Verification items for the finished model (mm, model axes). Face numbers are marked on the shaded views. A direction names the side the tool comes from. Coordinates: 2 decimals unless noted, no trailing zeros. Loops run counter-clockwise (first coordinate to the right, second up) from the corner with the lowest first, then second, coordinate; pieces in that order, holes last. Notation, with made-up numbers: (7, 43) - (28, 43) arc R20 cw to (28, 55) - close; hole circle Ø11 at (62.25, -39.75). An arc over 180 degrees is marked (long way). Answer as CSV lines item,"result". Start each with the question number.
1. Cross-section at C-C (z = -48). Enter the section's corners in (x, y) (3 decimals).
2. Set-up check for the marked faces 1 and 2: record each of +Z, -Z, +X, -X, +Y, -Y from which the full face is reachable in a straight line by a thin tool's end or side.
3. Gauge pin test, flat ends, axial feed: P1, Ø4, axis at y = 9, z = -36.5, coming from the -X side; P2, Ø3, axis at y = 14, z = -23.5, coming from the +X side; P3, Ø7.5, axis at y = 31, z = -40, coming from the +X side. Record the tip position at first contact, or that the pin passes through.
4. Cross-section at B-B (x = 13). Enter the section's corners in (y, z) (3 decimals).
5. Release check for a two-part mould opening along Y. For the marked faces 3, 4, 5 and 6 record: pulls with the +Y half, pulls with the -Y half, needs draft (parallel to the pull), parting line crosses it, or undercut.
6. Cross-section at D-D (x = 60). Enter the section's corners in (y, z) (3 decimals), plus the area to 3 significant figures.
7. Material ranges on line 1 (X direction, y = 3.5, z = -13.5) (3 decimals); line 2 (X direction, y = 24.5, z = -34) (3 decimals); line 3 (Y direction, x = 59.5, z = -27.5) (3 decimals), recorded low to high. Write a range as [from, to].
8. Cross-section at A-A (z = -28). Enter the section's corners in (x, y) (3 decimals).
```python
from build123d import *

# Parameters (mm, degrees)
SKETCH1_W           = 79.375
SKETCH1_H           = 57.14999999999999
BASE_EXTRUDE_DEPTH  = 9.525
SKETCH2_R           = 5.1562
CUT_EXTRUDE1_DEPTH  = 99.27125088244273
BOSS_EXTRUDE1_DEPTH = 11.112499999999999
FILLET1_R           = 4.7625
FILLET3_R           = 3.175
FILLET5_R           = 6.35
FILLET6_R           = 3.175


with BuildPart() as part:
    # Sketch1 → Base-Extrude (new body)
    with BuildSketch(Plane(origin=(0, 0, 0), x_dir=(1, 0, 0), z_dir=(0, 1, 0))):
        with Locations((39.6875, 28.574999999999996)):
            Rectangle(SKETCH1_W, SKETCH1_H)
    extrude(amount=BASE_EXTRUDE_DEPTH)

    # Sketch2 → Cut-Extrude1 (cut, through all)
    with BuildSketch(Plane(origin=(0, 9.525, 0), x_dir=(-1, 0, 0), z_dir=(0, 1, 0))):
        with Locations(Location((-11.112499999999999, -46.037499999999994, 0), (0, 0, 90))):
            Circle(SKETCH2_R)
        with Locations(Location((-11.112499999999999, -11.112499999999997, 0), (0, 0, 90))):
            Circle(SKETCH2_R)
        with Locations(Location((-68.2625, -11.112499999999997, 0), (0, 0, 90))):
            Circle(SKETCH2_R)
        with Locations(Location((-68.2625, -46.037499999999994, 0), (0, 0, 90))):
            Circle(SKETCH2_R)
    extrude(amount=-CUT_EXTRUDE1_DEPTH, mode=Mode.SUBTRACT)

    # Sketch3 → Boss-Extrude1 (add, symmetric)
    with BuildSketch(Plane(origin=(39.6875, 0, 0), x_dir=(0, 0, -1), z_dir=(1, 0, 0))):
        with BuildLine():
            Line((15.081249999999999, 9.525), (57.15, 9.525))
            Line((57.15, 9.525), (45.642080901347875, 34.2124833053063))
            ThreePointArc((45.642080901347875, 34.2124833053063), (40.65983135726152, 39.74024710013013), (33.435990911126424, 41.52773480629668))
            Line((33.435990911126424, 41.52773480629668), (24.475888920836205, 41.03647902618064))
            ThreePointArc((24.475888920836205, 41.03647902618064), (22.228971581677126, 38.79627321294108), (24.202681662531663, 36.31199703436931))
            Line((24.202681662531663, 36.31199703436931), (28.991955012405008, 35.48840889689211))
            ThreePointArc((28.991955012405008, 35.48840889689211), (34.924994788062534, 28.439370658797703), (28.97494247235726, 21.40468669276046))
            Line((28.97494247235726, 21.40468669276046), (17.72572001228568, 19.498181673786302))
            ThreePointArc((17.72572001228568, 19.498181673786302), (15.830857484241669, 18.416745811263993), (15.081249999999997, 16.367820203902035))
            Line((15.081249999999997, 16.367820203902035), (15.081249999999999, 9.525))
        make_face()
    extrude(amount=BOSS_EXTRUDE1_DEPTH, both=True)

    # Fillet1
    fillet1_edges = [part.edges().sort_by_distance(p)[0] for p in [
        (0, 4.7625, -57.15),
        (79.375, 4.7625, -57.15),
        (79.375, 4.7625, 0),
        (0, 4.7625, 0),
    ]]
    fillet(fillet1_edges, radius=FILLET1_R)

    # Fillet3
    fillet3_edges = [part.edges().sort_by_distance(p)[0] for p in [
        (16.668750000000003, 9.525, -57.15),
        (39.6875, 9.525, 0),
        (0, 9.525, -28.575),
        (79.375, 9.525, -28.575),
        (62.70625, 9.525, -57.15),
        (77.98009604540093, 9.525, -55.75509604540093),
        (1.3949039545990662, 9.525, -55.75509604540093),
        (77.98009604540093, 9.525, -1.3949039545990662),
        (1.3949039545990667, 9.525, -1.3949039545990662),
    ]]
    fillet(fillet3_edges, radius=FILLET3_R)

    # Fillet5
    # the kernel refuses this fillet: 6.35 mm, written as the material it adds along each edge
    with BuildSketch(Plane(origin=(28.575000000000003, 9.525, -15.081249999999997), x_dir=(-1, 0, 0), z_dir=(0, 0, -1))) as fillet5_piece_1:
        with BuildLine():
            CenterArc((FILLET5_R, FILLET5_R), FILLET5_R, 180, 90)
            Line((0, FILLET5_R), (0, 0))
            Line((0, 0), (FILLET5_R, 0))
        make_face()
    extrude(amount=38.893750000000004)
    with BuildSketch(Plane(origin=(50.8, 9.525, -15.081249999999999), x_dir=(0, 0, 1), z_dir=(-1, 0, 0))) as fillet5_piece_2:
        with BuildLine():
            CenterArc((FILLET5_R, FILLET5_R), FILLET5_R, 180, 90)
            Line((3.55e-15, FILLET5_R), (0, 0))
            Line((0, 0), (FILLET5_R, 0))
        make_face()
    extrude(amount=22.224999999999994)
    with BuildSketch(Plane(origin=(50.8, 9.525, -15.081249999999997), x_dir=(1, 0, 0), z_dir=(0, 0, -1))) as fillet5_piece_3:
        with BuildLine():
            CenterArc((FILLET5_R, -FILLET5_R), FILLET5_R, 90, 90)
            Line((0, -FILLET5_R), (0, 0))
            Line((0, 0), (FILLET5_R, 0))
        make_face()
    extrude(amount=38.893750000000004)
    with BuildSketch(Plane(origin=(28.575000000000003, 6.350000000000001, -53.975), x_dir=(0, 1, 0), z_dir=(0, 0, 1))) as fillet5_piece_4_section:
        with BuildLine():
            CenterArc((3.174999999999999 + FILLET5_R, FILLET5_R), FILLET5_R, 180.00000000000003, 90)
            Line((3.174999999999999, FILLET5_R), (3.174999999999999, 0))
            Line((3.174999999999999, 0), (3.174999999999999 + FILLET5_R, 0))
        make_face()
    fillet5_piece_4 = revolve(axis=Axis((28.575000000000003, 6.350000000000001, -53.975), (-1, 0, 0)), revolution_arc=359.64000000000004, mode=Mode.PRIVATE)
    fillet5_piece_4 = split(fillet5_piece_4, bisect_by=Plane(origin=(28.575000000000003, 0, -53.975), z_dir=(0, 1, 0)), keep=Keep.TOP, mode=Mode.PRIVATE)
    fillet5_piece_4 = split(fillet5_piece_4, bisect_by=Plane(origin=(28.575000000000003, 6.350000000000001, -57.15), z_dir=(0, 0, 1)), keep=Keep.TOP, mode=Mode.PRIVATE)
    fillet5_piece_4 = split(fillet5_piece_4, bisect_by=Plane(origin=(28.575000000000003, 8.132568412888961, -57.799073453811204), z_dir=(0, -0.42249632325246483, 0.9063646379014071)), keep=Keep.TOP, mode=Mode.PRIVATE)
    add(fillet5_piece_4)
    with BuildSketch(Plane(origin=(50.8, 6.350000000000001, -53.975), x_dir=(0, 1, 0), z_dir=(0, 0, 1))) as fillet5_piece_5_section:
        with BuildLine():
            CenterArc((3.174999999999999 + FILLET5_R, -FILLET5_R), FILLET5_R, 90, 90)
            Line((3.174999999999999, -FILLET5_R), (3.174999999999999, 0))
            Line((3.174999999999999, 0), (3.174999999999999 + FILLET5_R, 0))
        make_face()
    fillet5_piece_5 = revolve(axis=Axis((50.8, 6.350000000000001, -53.975), (-1, 0, 0)), revolution_arc=359.64000000000004, mode=Mode.PRIVATE)
    fillet5_piece_5 = split(fillet5_piece_5, bisect_by=Plane(origin=(50.8, 0, -53.975), z_dir=(0, 1, 0)), keep=Keep.TOP, mode=Mode.PRIVATE)
    fillet5_piece_5 = split(fillet5_piece_5, bisect_by=Plane(origin=(50.8, 6.350000000000001, -57.15), z_dir=(0, 0, 1)), keep=Keep.TOP, mode=Mode.PRIVATE)
    fillet5_piece_5 = split(fillet5_piece_5, bisect_by=Plane(origin=(50.8, 8.132568412888961, -57.799073453811204), z_dir=(0, -0.42249632325246483, 0.9063646379014071)), keep=Keep.TOP, mode=Mode.PRIVATE)
    add(fillet5_piece_5)
    with BuildSketch(Plane(origin=(28.575000000000003, 9.525, 0.7937500000000028), x_dir=(-1, 0, 0), z_dir=(0, 0, -1))) as fillet5_piece_6a_section:
        with BuildLine():
            CenterArc((FILLET5_R, FILLET5_R), FILLET5_R, 180, 90)
            Line((0, FILLET5_R), (0, 0))
            Line((0, 0), (FILLET5_R, 0))
        make_face()
    fillet5_piece_6a = extrude(amount=54.768750000000004, mode=Mode.PRIVATE)
    fillet5_piece_6a = split(fillet5_piece_6a, bisect_by=Plane(origin=(28.575000000000003, 9.525000000000004, -15.081249999999999), z_dir=(0, -2.6e-16, 1)), keep=Keep.TOP, mode=Mode.PRIVATE)
    with BuildSketch(Plane(origin=(50.8, 9.525, -15.081249999999999), x_dir=(0, 0, 1), z_dir=(-1, 0, 0))) as fillet5_piece_6b_section:
        with BuildLine():
            CenterArc((FILLET5_R, FILLET5_R), FILLET5_R, 180, 90)
            Line((3.55e-15, FILLET5_R), (0, 0))
            Line((0, 0), (FILLET5_R, 0))
        make_face()
    fillet5_piece_6b = extrude(amount=38.1, mode=Mode.PRIVATE)
    fillet5_piece_6b = fillet5_piece_6b - Plane(origin=(11.112499999999999, 9.525, -11.112499999999997), x_dir=(-6e-17, 0, 1), z_dir=(0, 1, 0)) * Cylinder(5.1562, 102, mode=Mode.PRIVATE)
    fillet5_piece_6b = split(fillet5_piece_6b, bisect_by=Plane(origin=(28.575000000000003, 9.525, -15.081249999999999), z_dir=(-1, 0, 0)), keep=Keep.TOP, mode=Mode.PRIVATE)
    fillet5_piece_6 = fillet5_piece_6a & fillet5_piece_6b
    add(fillet5_piece_6)
    with BuildSketch(Plane(origin=(66.675, 9.525, -15.081249999999999), x_dir=(0, 0, 1), z_dir=(-1, 0, 0))) as fillet5_piece_7a_section:
        with BuildLine():
            CenterArc((FILLET5_R, FILLET5_R), FILLET5_R, 180, 90)
            Line((3.55e-15, FILLET5_R), (0, 0))
            Line((0, 0), (FILLET5_R, 0))
        make_face()
    fillet5_piece_7a = extrude(amount=38.099999999999994, mode=Mode.PRIVATE)
    fillet5_piece_7a = fillet5_piece_7a - Plane(origin=(68.2625, 9.525, -11.112499999999997), x_dir=(-6e-17, 0, 1), z_dir=(0, 1, 0)) * Cylinder(5.1562, 102, mode=Mode.PRIVATE)
    fillet5_piece_7a = split(fillet5_piece_7a, bisect_by=Plane(origin=(50.8, 9.525, -15.081249999999999), z_dir=(1, 0, 0)), keep=Keep.TOP, mode=Mode.PRIVATE)
    with BuildSketch(Plane(origin=(50.8, 9.525, 0.7937500000000028), x_dir=(1, 0, 0), z_dir=(0, 0, -1))) as fillet5_piece_7b_section:
        with BuildLine():
            CenterArc((FILLET5_R, -FILLET5_R), FILLET5_R, 90, 90)
            Line((0, -FILLET5_R), (0, 0))
            Line((0, 0), (FILLET5_R, 0))
        make_face()
    fillet5_piece_7b = extrude(amount=54.768750000000004, mode=Mode.PRIVATE)
    fillet5_piece_7b = split(fillet5_piece_7b, bisect_by=Plane(origin=(50.8, 9.525000000000004, -15.081249999999999), z_dir=(0, -2.6e-16, 1)), keep=Keep.TOP, mode=Mode.PRIVATE)
    fillet5_piece_7 = fillet5_piece_7a & fillet5_piece_7b
    add(fillet5_piece_7)

    # Fillet6
    fillet6_edges = [part.edges().sort_by_distance(p)[0] for p in [
        (39.6875, 9.525000000000507, -57.150000000000006),
    ]]
    fillet(fillet6_edges, radius=FILLET6_R)


solid = part.part
```
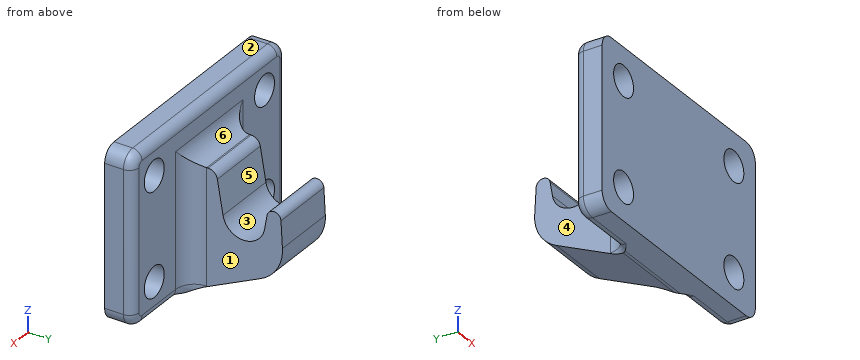
Values follow:
1,outline,"(0, 0) - (6.344, 0) - (6.344, 9.525) - (3.175, 9.525) arc R3.175 ccw to (0, 6.35) - close; (15.881, 0) - (63.494, 0) - (63.494, 9.525) - (57.15, 9.525) arc R6.35 cw to (50.8, 15.875) - (50.8, 29.154) - (28.575, 29.154) - (28.575, 15.875) arc R6.35 cw to (22.225, 9.525) - (15.881, 9.525) - close; (73.031, 0) - (79.375, 0) - (79.375, 6.35) arc R3.175 ccw to (76.2, 9.525) - (73.031, 9.525) - close"
2,face 1,"+Z, -Z, +X, +Y"
2,face 2,"+Z, +X, -X, +Y, -Y"
3,P1,"stops at x = 0.07"
3,P2,"stops at x = 51.77"
3,P3,"stops at x = 50.8"
4,outline,"(0, -57.15) - (6.35, -57.15) arc R3.175 ccw to (9.525, -53.975) - (9.525, -50.836) - (0, -50.836) - close; (0, -41.239) - (9.525, -41.239) - (9.525, -15.911) - (0, -15.911) - close; (0, -6.314) - (9.525, -6.314) - (9.525, -3.175) arc R3.175 ccw to (6.35, 0) - (0, 0) - close"
5,face 3,"undercut"
5,face 4,"needs draft"
5,face 5,"undercut"
5,face 6,"pulls with the +Y half"
6,outline,"(0, -57.15) - (6.35, -57.15) arc R3.175 ccw to (9.525, -53.975) - (9.525, -3.175) arc R3.175 ccw to (6.35, 0) - (0, 0) - close"
6,area,"540 mm²"
7,line 1,"x = [0, 6.542], [15.683, 63.692], [72.833, 79.375]"
7,line 2,"x = [28.575, 50.8]"
7,line 3,"y = [0, 9.525]"
8,outline,"(0, 0) - (79.375, 0) - (79.375, 6.35) arc R3.175 ccw to (76.2, 9.525) - (57.15, 9.525) arc R6.35 cw to (50.8, 15.875) - (50.8, 21.239) - (28.575, 21.239) - (28.575, 15.875) arc R6.35 cw to (22.225, 9.525) - (3.175, 9.525) arc R3.175 ccw to (0, 6.35) - close; (28.575, 35.659) - (50.8, 35.659) - (50.8, 41.23) - (28.575, 41.23) - close"
